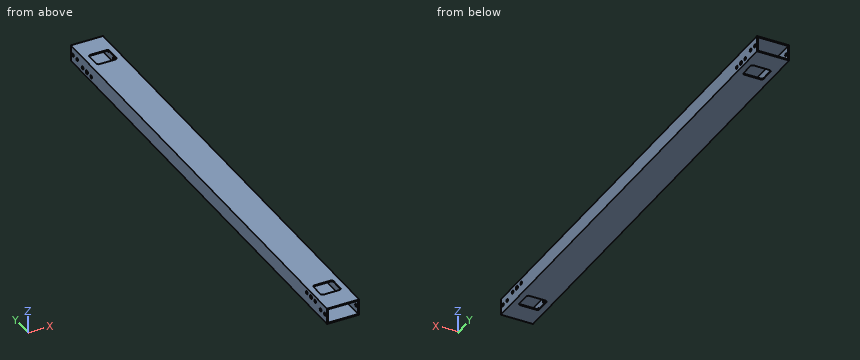
```python
from build123d import *

# Parameters (mm, degrees)
SKETCH1_W               = 50.8
SKETCH1_H               = 762
BOSS_EXTRUDE1_DEPTH     = 12.7
SHELL1_T                = -1.5875
SKETCH3_R               = 2.4892
CUT_EXTRUDE1_DEPTH      = 383.056867495
CUT_EXTRUDE2_DEPTH      = 383.056867495
CUT_EXTRUDE2_DEPTH_BACK = 383.056867495
SKETCH4_R               = 3.175
SKETCH4_R_2             = 2.4892
CUT_EXTRUDE4_DEPTH      = 383.056867495
CUT_EXTRUDE4_DEPTH_BACK = 383.056867495
SKETCH5_W               = 31.75
SKETCH5_H               = 26.9875
FILLET1_R               = 3.175


with BuildPart() as part:
    # Sketch1 → Boss-Extrude1 (new, symmetric)
    with BuildSketch(Plane.XY):
        Rectangle(SKETCH1_W, SKETCH1_H)
    extrude(amount=BOSS_EXTRUDE1_DEPTH, both=True)

    # Shell1
    shell1_openings = [part.faces().sort_by_distance(p)[0] for p in [
        (0, -381, 0),
        (0, 381, 0),
    ]]
    offset(amount=SHELL1_T, openings=shell1_openings, kind=Kind.INTERSECTION)

    # Sketch3 → Cut-Extrude1 (cut, symmetric)
    with BuildSketch(Plane(origin=(0, 0, 0), x_dir=(0, 0, -1), z_dir=(1, 0, 0))):
        with Locations((0, -374.65)):
            Circle(SKETCH3_R)
        with Locations((0, -361.95)):
            Circle(SKETCH3_R)
    cut_extrude1 = extrude(amount=CUT_EXTRUDE1_DEPTH, both=True, mode=Mode.SUBTRACT)

    # Sketch4 → Cut-Extrude2 (cut, two sides: drawn at the far end of the back side and taken through both)
    with BuildSketch(Plane(origin=(0, 0, 0), x_dir=(0, 0, -1), z_dir=(1, 0, 0)).offset(-CUT_EXTRUDE2_DEPTH_BACK)):
        with Locations((4.7625, 333.375)):
            Circle(SKETCH4_R)
        with Locations((4.7625, 346.075)):
            Circle(SKETCH4_R_2)
        with Locations((4.7625, 320.675)):
            Circle(SKETCH4_R_2)
        with Locations((-4.7625, -333.375)):
            Circle(SKETCH4_R)
        with Locations((-4.7625, -320.675)):
            Circle(SKETCH4_R_2)
        with Locations((-4.7625, -346.075)):
            Circle(SKETCH4_R_2)
    extrude(amount=CUT_EXTRUDE2_DEPTH + CUT_EXTRUDE2_DEPTH_BACK, mode=Mode.SUBTRACT)

    # Mirror1: Cut-Extrude1 across plane
    add(cut_extrude1.mirror(Plane.ZX), mode=Mode.SUBTRACT)

    # Sketch5 → Cut-Extrude4 (cut, two sides: drawn at the far end of the back side and taken through both)
    with BuildSketch(Plane.XY.offset(-CUT_EXTRUDE4_DEPTH_BACK)):
        with Locations((0, -333.375)):
            Rectangle(SKETCH5_W, SKETCH5_H)
        with Locations((0, 333.375)):
            Rectangle(SKETCH5_W, SKETCH5_H)
    extrude(amount=CUT_EXTRUDE4_DEPTH + CUT_EXTRUDE4_DEPTH_BACK, mode=Mode.SUBTRACT)

    # Fillet1
    fillet1_edges = [part.edges().sort_by_distance(p)[0] for p in [
        (-15.875, -346.86875, -11.90625),
        (-15.875, -319.88125, -11.90625),
        (15.875, -319.88125, -11.90625),
        (15.875, -346.86875, -11.90625),
        (-15.875, -346.86875, 11.90625),
        (-15.875, -319.88125, 11.90625),
        (15.875, -319.88125, 11.90625),
        (15.875, -346.86875, 11.90625),
        (15.875, 319.88125, -11.90625),
        (-15.875, 319.88125, -11.90625),
        (-15.875, 346.86875, -11.90625),
        (15.875, 346.86875, -11.90625),
        (15.875, 319.88125, 11.90625),
        (-15.875, 319.88125, 11.90625),
        (-15.875, 346.86875, 11.90625),
        (15.875, 346.86875, 11.90625),
    ]]
    fillet(fillet1_edges, radius=FILLET1_R)


solid = part.part
```
Build history of the part. All positions in model axes, mm. Round coordinates to 2 decimals unless told otherwise and drop trailing zeros. Write each loop counter-clockwise with the first axis right and the second up, starting at its lowest first coordinate (ties: lowest second). Pieces come first, ordered by that corner, then holes. Notation, with made-up numbers: (-15, -36) -> (33, -36) arc R20 cw to (33, -4) -> close; hole circle Ø4 at (-18, -11). An arc over 180 degrees is marked (long way). Put each result on its own line as item: value.
Item 1: Flat gauge pin, fed straight in: P1, Ø5.5, axis at y = 374.65, z = 0, coming from the +X side. Where does the tip first touch, or does it go through?
Here are the results:
P1: stops at x = 25.4
Item 2: Wall check: probe 1 along Y at (x, z) = (0, 11.5); probe 2 along Y at (x, z) = (-24.5, 0); probe 3 along X at (y, z) = (138, 7). Give the ranges that are in metal, low to high. Write a range as from..to.
Here are the results:
probe 1: y = -381..-346.87, -319.88..319.88, 346.87..381
probe 2: y = -381..-377.14, -372.16..-364.44, -359.46..359.46, 364.44..372.16, 377.14..381
probe 3: x = -25.4..-23.81, 23.81..25.4
Item 3: Slice it at A-A, the plane y = 234. Give the cut face in (x, z), plus the area to 3 significant figures.
Here are the results:
outline: (-25.4, -12.7) -> (25.4, -12.7) -> (25.4, 12.7) -> (-25.4, 12.7) -> close; hole (-23.81, -11.11) -> (23.81, -11.11) -> (23.81, 11.11) -> (-23.81, 11.11) -> close
area: 232 mm^2
